The listing builds one solid part. Answer for the finished solid, in the listing's coordinates (mm). A direction names the side the tool comes from. Round coordinates to 2 decimals unless told otherwise and drop trailing zeros. Write each loop counter-clockwise with the first axis right and the second up, starting at its lowest first coordinate (ties: lowest second). Pieces come first, ordered by that corner, then holes. Notation, with made-up numbers: M 37.5,13 L 93.5,13 A28 cw 93.5,31 Z; hole C 78,23.25 d3. An arc over 180 degrees is marked long. One line per item, written item: value. Start each with the question number.
(1) Section C-C (y = -11.25) is taken. Determine the outline of the cut face in (x, z), plus the area to 3 significant figures.
(2) Given P1, Ø1.5, axis at x = 19.5, z = -4.5, coming from the +Y side; P2, Ø4, axis at x = -11, y = -13, coming from the +Z side; P3, Ø4, axis at y = -19.5, z = 44, coming from the +X side; P4, Ø2, axis at x = 11.5, z = 35.5, coming from the -Y side, each flat-ended and moving along its own axis, determine where each tip first touches the part or whether it passes through.
(3) For faces 4 (the flat face through (14.9, -18.4, 55)), 5 (the flat face through (14, -14, 15)), 6 (the flat face through (-15, -15, 15)), determine the directions among +Z, -Z, +X, -X, +Y, -Y from which every point of the face is accessible in a straight line to the end or side of a thin tool.
(4) For a pull along X with two mould halves and no side action, classify faces 1 (the flat face through (26.523, -14.79, 34.72)), 2 (the cylindrical face through (18.46, -15.3, 35.28)), 3 (the flat face through (0, -30, 0)) as released by +X, released by -X, zero draft, split by the parting line, or undercut.
(5) Section D-D (z = 51) is taken. Determine the outline of the cut face in (x, y), plus the area to 3 significant figures.
(6) Section A-A (x = 12) is taken. Determine the outline of the cut face in (y, z), plus the area to 3 significant figures.
(7) Section B-B (z = 41) is taken. Determine the outline of the cut face in (x, y), plus the area to 3 significant figures.
(8) Consider probe 1 along Z at (x, y) = (-5.5, -27.25); probe 2 along X at (y, z) = (-11, 16.5); probe 3 along Y at (x, z) = (11, 43.5). Determine where each line is inside the solid, lowest interval first.
```python
from build123d import *

# Parameters (mm, degrees)
F0_W     = 60
F0_H     = 30
F1_DEPTH = 30
F2_W     = 30
F2_H     = 30
F3_DEPTH = 40
F3_TAPER = 10
F4_R     = 4.2494021433
F5_DEPTH = 40


with BuildPart() as f1:
    # F0 (on Front) → F1 (new body)
    with BuildSketch(Plane.XZ):
        Rectangle(F0_W, F0_H)
    extrude(amount=F1_DEPTH)

    # F2 (on face) → F3 (join)
    with BuildSketch(Plane.XY.offset(15)):
        with Locations((15, -15)):
            Rectangle(F2_W, F2_H)
    extrude(amount=F3_DEPTH, taper=F3_TAPER)

    # F4 (on face) → F5 (cut)
    with BuildSketch(Plane.XY.offset(55)):
        with Locations((14.5341921598, -13.6707741767)):
            Circle(F4_R)
    extrude(amount=-F5_DEPTH, mode=Mode.SUBTRACT)


solid = f1.part
```
Recorded:
1. outline: M -30,-15 L 30,-15 L 30,15 L 22.95,55 L 18.03,55 L 18.03,15 L 11.04,15 L 11.04,55 L 7.05,55 L 0,15 L -30,15 Z
1. area: 2,440 mm2
2. P1: stops at y = 0
2. P2: stops at z = 15
2. P3: stops at x = 25.24
2. P4: stops at y = -26.56
3. face 4: +Z, +X, -X, +Y, -Y
3. face 5: +Z
3. face 6: +Z, -X, +Y, -Y
4. face 1: released by +X
4. face 2: undercut
4. face 3: zero draft
5. outline: M 6.35,-23.65 L 23.65,-23.65 L 23.65,-6.35 L 6.35,-6.35 Z; hole C 14.53,-13.67 d8.5
5. area: 243 mm2
6. outline: M -30,-15 L 0,-15 L 0,15 L -7.05,55 L -10.26,55 L -10.26,15 L -17.08,15 L -17.08,55 L -22.95,55 L -30,15 Z
6. area: 1,540 mm2
7. outline: M 4.58,-25.42 L 25.42,-25.42 L 25.42,-4.58 L 4.58,-4.58 Z; hole C 14.53,-13.67 d8.5
7. area: 377 mm2
8. probe 1: z = -15 to 15
8. probe 2: x = 0.26 to 11.23, 17.84 to 29.74
8. probe 3: y = -24.97 to -16.03, -11.31 to -5.03
